```python
from build123d import *

# Parameters (mm, degrees)
MODEL_R                 = 1.5
SALIENTE_EXTRUIR1_DEPTH = 3


with BuildPart() as part:
    # Model → Saliente-Extruir1 (new body)
    with BuildSketch(Plane.XY):
        with BuildLine():
            Line((213.25077615, 80.428489513), (213.25077615, 188.428489513))
            ThreePointArc((213.25077615, 188.428489513), (208.75077615, 192.928489513), (204.25077615, 188.428489513))
            Line((204.25077615, 188.428489513), (204.25077615, 80.428489513))
            ThreePointArc((204.25077615, 80.428489513), (208.75077615, 75.928489513), (213.25077615, 80.428489513))
        make_face()
        with Locations((208.75077615, 179.428489513)):
            Circle(MODEL_R, mode=Mode.SUBTRACT)
        with Locations((208.75077615, 188.428489513)):
            Circle(MODEL_R, mode=Mode.SUBTRACT)
        with Locations((208.75077615, 152.428489513)):
            Circle(MODEL_R, mode=Mode.SUBTRACT)
        with Locations((208.75077615, 161.428489513)):
            Circle(MODEL_R, mode=Mode.SUBTRACT)
        with Locations((208.75077615, 170.428489513)):
            Circle(MODEL_R, mode=Mode.SUBTRACT)
        with Locations((208.75077615, 143.428489513)):
            Circle(MODEL_R, mode=Mode.SUBTRACT)
        with Locations((208.75077615, 116.428489513)):
            Circle(MODEL_R, mode=Mode.SUBTRACT)
        with Locations((208.75077615, 125.428489513)):
            Circle(MODEL_R, mode=Mode.SUBTRACT)
        with Locations((208.75077615, 134.428489513)):
            Circle(MODEL_R, mode=Mode.SUBTRACT)
        with Locations((208.75077615, 80.428489513)):
            Circle(MODEL_R, mode=Mode.SUBTRACT)
        with Locations((208.75077615, 89.428489513)):
            Circle(MODEL_R, mode=Mode.SUBTRACT)
        with Locations((208.75077615, 98.428489513)):
            Circle(MODEL_R, mode=Mode.SUBTRACT)
        with Locations((208.75077615, 107.428489513)):
            Circle(MODEL_R, mode=Mode.SUBTRACT)
    extrude(amount=SALIENTE_EXTRUIR1_DEPTH)


solid = part.part
```
Verification items for the finished model (mm, model axes). Give positions to 0.01 mm unless a question says otherwise; leave off trailing zeros.
1. Mould release check, pull along Y, two halves, no side actions. Record for faces 1 (the flat face through (207, 135, 3)), 2 (the cylindrical face through (208.556, 189.916, 1.479)), 3 (the cylindrical face through (208.85, 192.927, 1.479)), 4 (the cylindrical face through (207.645, 135.442, 1.479)): released by +Y, released by -Y, zero draft, split by the parting line, or undercut.
2. Thickness scan on line 1 (X direction, y = 107, z = 0.85); line 2 (Y direction, x = 211.5, z = 1.35); line 3 (Y direction, x = 206.5, z = 0.8). Record the ranges inside material, lowest first.
3. Section check A-A, the plane z = 0.5. Count the separate pieces of the cut face and the enclosed holes in it, then the cut area to 3 significant figures.
4. Go/stop test with flat-tipped pins: pin 1 Ø4 at (x, y) = (208.75, 188.43) entering from +Z; pin 2 Ø2.5 at (x, y) = (208.75, 125.43) entering from +Z. Record where each tip stops, or that it passes through.
Geometry says:
1. face 1: zero draft
1. face 2: undercut
1. face 3: released by +Y
1. face 4: undercut
2. line 1: x = 204.25 to 207.31, 210.19 to 213.25
2. line 2: y = 76.87 to 191.99
2. line 3: y = 76.53 to 192.33
3. separate pieces: 1
3. enclosed holes: 13
3. area: 944 mm2
4. pin 1: stops at z = 3
4. pin 2: passes through
